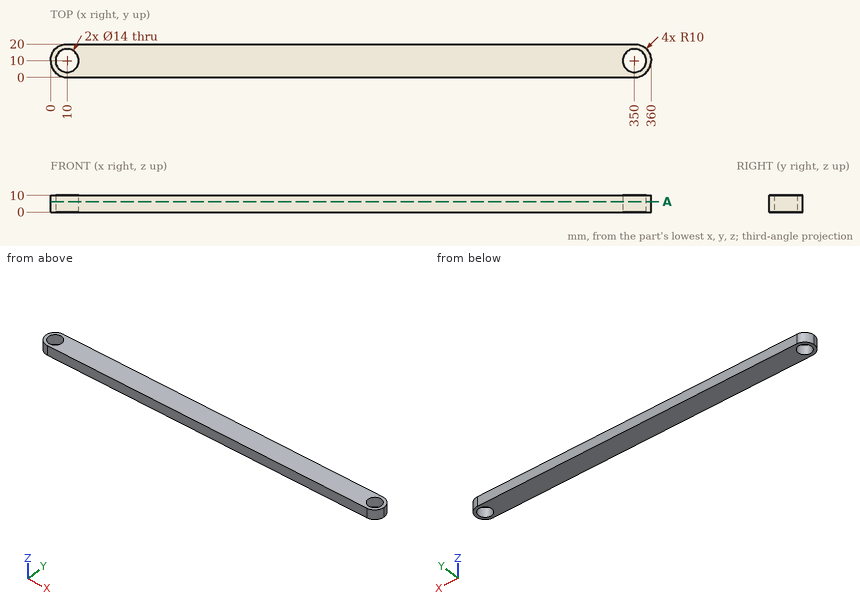
Verification items for this drawing (mm, ordinates from the low corner). Coordinates: 2 decimals unless noted, no trailing zeros. Answer in a Markdown table with one row per item. Add a question column.
1. Material ranges on L1, parallel to Y at x = 10, z = 6.25; L2, parallel to X at y = 7.25, z = 1.25; L3, parallel to X at y = 11.5, z = 7.5, recorded low to high. Write a range as [from, to].
2. Section check A-A (z = 6.25). Give the number of separate pieces and of enclosed holes in the cut face, plus the area to 3 significant figures.
3. Gauge pin test, flat ends, axial feed: pin 1 Ø6 at (y, z) = (3.5, 7.5) entering from +X; pin 2 Ø2 at (y, z) = (12.5, 3) entering from -X. Record the tip position at first contact, or that the pin passes through.
Data:
| question | item | result |
|---|---|---|
| 1 | L1 | y = [0, 3], [17, 20] |
| 1 | L2 | x = [0.39, 3.56], [16.44, 343.56], [356.44, 359.61] |
| 1 | L3 | x = [0.11, 3.16], [16.84, 343.16], [356.84, 359.89] |
| 2 | separate pieces | 1 |
| 2 | enclosed holes | 2 |
| 2 | area | 6,810 mm² |
| 3 | pin 1 | stops at x = 359.37 |
| 3 | pin 2 | stops at x = 0.11 |
